from build123d import *

# Parameters (mm, degrees)
F2_T     = -3.175
F4_DEPTH = 1.5875


with BuildPart() as f1:
    # F0 (on Front) → F1 (revolve)
    with BuildSketch(Plane.XZ):
        Polygon((-38.1, 0), (0, 0), (0, 159.4304591417), (-62.6866146922, 159.4304591417), align=None)
    revolve(axis=Axis((0, 0, 79.7152295709), (0, 0, -1)))

    # F2
    f2_openings = [f1.faces().sort_by_distance(p)[0] for p in [
        (0, 0, 159.430459),
    ]]
    offset(amount=F2_T, openings=f2_openings)

    # F3 (on Top) → F4 (cut)
    with BuildSketch(Plane.XY):
        with BuildLine():
            add(Edge.make_bspline(
                [(-19.4014832377, 4.2113135569), (-18.7531898055, 5.4777192579), (-17.4014889021, 8.1181929151), (-12.5510655032, 10.5482010959), (-9.3620261804, 10.190664987), (-7.7923568897, 10.0146830082)],
                knots=[0, 0, 0, 0, 0.318803598, 0.6647099753, 1, 1, 1, 1], degree=3))
            add(Edge.make_bspline(
                [(-7.7923568897, 10.0146830082), (-7.9133892647, 7.7789314659), (-8.1642059751, 3.1457591674), (-9.4585773774, -4.4941025574), (-12.891941134, -12.5420703822), (-17.5861383279, -16.7926160144), (-17.5102852366, -20.7671425935), (-16.4796150747, -22.6430773976), (-14.8305156939, -23.8501410331), (-12.9807029748, -24.2714401619), (-10.5467395482, -23.8279743211), (-8.4582492729, -22.2675558352), (-6.1108322547, -16.5517126321), (-5.438963665, -7.3460077185), (-4.4365950396, 3.6569436415), (-3.853734117, 10.0549794734)],
                knots=[0, 0, 0, 0, 0.0880409595, 0.1824482404, 0.2824178019, 0.3656698949, 0.4286344499, 0.4769656385, 0.5238340761, 0.5699241603, 0.6214860687, 0.6740104117, 0.754350396, 0.8571587825, 1, 1, 1, 1], degree=3))
            add(Edge.make_bspline(
                [(-3.853734117, 10.0549794734), (-0.6908265253, 10.0549794734), (2.4720810664, 10.0549794734), (5.6349886581, 10.0549794734)],
                knots=[0, 0, 0, 0, 9.4887227751, 9.4887227751, 9.4887227751, 9.4887227751], degree=3))
            add(Edge.make_bspline(
                [(5.6349886581, 10.0549794734), (5.1179656529, 4.2988011186), (4.1855989826, -6.0815277883), (2.2418363662, -17.133074814), (6.1993286809, -22.8137367886), (9.6258734077, -24.3046887574), (12.8862283177, -24.0371426728), (15.1074594417, -23.8919320147), (19.0561707704, -20.2535401147), (20.3748776318, -17.2807457035), (21.0926160049, -12.3105993929), (21.1163228045, -12.2759174556)],
                knots=[0, 0, 0, 0, 0.1918449829, 0.3459611394, 0.461688353, 0.5500217309, 0.6322196488, 0.7017930408, 0.8051710251, 0.9007838703, 0.9983000374, 0.9983000374, 0.9983000374, 0.9983000374], degree=3))
            add(Edge.make_bspline(
                [(21.1163228045, -12.2759174556), (20.3916681002, -12.2759174556), (19.6672989739, -12.2759174556), (19.5691268891, -12.2759174556)],
                knots=[0.0004126536, 0.0004126536, 0.0004126536, 0.0004126536, 0.9048401528, 0.9048401528, 0.9048401528, 0.9048401528], degree=3))
            add(Edge.make_bspline(
                [(19.5691268891, -12.2759174556), (19.418191644, -13.2654511474), (19.1064893287, -15.3089761217), (16.123951194, -17.5847200897), (13.3802481357, -17.4290693932), (9.9866685411, -15.0695037941), (9.2467731261, -8.3072976675), (10.5787837329, 1.0040330336), (11.1519221552, 7.0625804664), (11.4350030199, 10.0549794734)],
                knots=[0, 0, 0, 0, 0.1099798537, 0.2271237245, 0.3287414252, 0.4492038413, 0.610060749, 0.8074036986, 1, 1, 1, 1], degree=3))
            add(Edge.make_bspline(
                [(11.4350030199, 10.0549794734), (14.6624402454, 10.0549794734), (17.8898774708, 10.0549794734), (21.1173146963, 10.0549794734)],
                knots=[0, 0, 0, 0, 9.6823116764, 9.6823116764, 9.6823116764, 9.6823116764], degree=3))
            add(Edge.make_bspline(
                [(21.1173146963, 10.0549794734), (21.1173146963, 12.1795317779), (21.1173146963, 14.3040840824), (21.1173146963, 16.428636387)],
                knots=[0, 0, 0, 0, 6.3736569136, 6.3736569136, 6.3736569136, 6.3736569136], degree=3))
            add(Edge.make_bspline(
                [(21.1173146963, 16.428636387), (10.6683538258, 16.5466721162), (-5.2496723323, 16.7264886403), (-13.2144965635, 15.9136449775), (-17.6553820034, 13.2925715926), (-19.0221552591, 8.7173019267), (-20.1733487063, 5.7306348498), (-20.7589622587, 4.2113135569)],
                knots=[0, 0, 0, 0, 0.3620561729, 0.551559117, 0.6983516808, 0.8465511212, 1, 1, 1, 1], degree=3))
            add(Edge.make_bspline(
                [(-20.7589622587, 4.2113135569), (-20.3064692517, 4.2113135569), (-19.8539762447, 4.2113135569), (-19.4014832377, 4.2113135569)],
                knots=[0, 0, 0, 0, 1.357479021, 1.357479021, 1.357479021, 1.357479021], degree=3))
        make_face()
    extrude(amount=F4_DEPTH, mode=Mode.SUBTRACT)


solid = f1.part
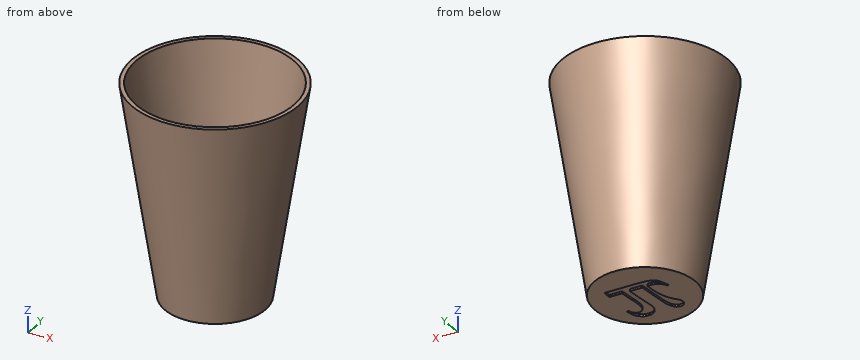
For this review, take the finished solid that the model builds, in its own axes (mm). Coordinates: 2 decimals unless noted, no trailing zeros. Write each loop counter-clockwise with the first axis right and the second up, starting at its lowest first coordinate (ties: lowest second). Pieces come first, ordered by that corner, then holes. Notation, with made-up numbers: (10.25, 40) -> (54.25, 40) arc R11 cw to (54.25, 48) -> close; hole circle Ø3 at (16.25, 86.5). An arc over 180 degrees is marked (long way). Write each question's results on one line, items separated by ' | '. Start each with the question number.
1) Consider section B-B (z = 143). Write out the cut boundary in (x, y), plus the area to 3 significant figures.
2) Insertion check: pin 1 (2 mm diameter, centred on x = -22.5, y = 8, fed in from +Z) (3 decimals); pin 2 (1.5 mm diameter, centred on x = 43, z = 113.5, fed in from -Y); pin 3 (4 mm diameter, centred on y = 22.5, z = 131.5, fed in from -X). Each pin has a flat end and moves straight along its axis. Give the tip position at first contact, or say it passes through.
3) Consider section A-A (z = 110). Write out the cut boundary in (x, y), plus the area to 3 significant figures.
4) Wall thickness on L1, parallel to Y at x = -42.5, z = 93; L2, parallel to Z at x = -31, y = -13.5 (3 decimals); L3, parallel to X at y = 7.5, z = 64.5: over which ranges is each line inside the solid? List them lowest first. Write a range as [from, to].
Geometry says:
1) outline: circle Ø120.31 at (0, 0); hole circle Ø113.88 at (0, 0) | area: 1,180 mm^2
2) pin 1: z = 3.175 | pin 2: y = -36.17 | pin 3: x = -54.73
3) outline: circle Ø110.13 at (0, 0); hole circle Ø103.7 at (0, 0) | area: 1,080 mm^2
4) L1: [-30.72, -24.85], [24.85, 30.72] | L2: [0, 3.175] | L3: [-47.46, -44.2], [44.2, 47.46]
